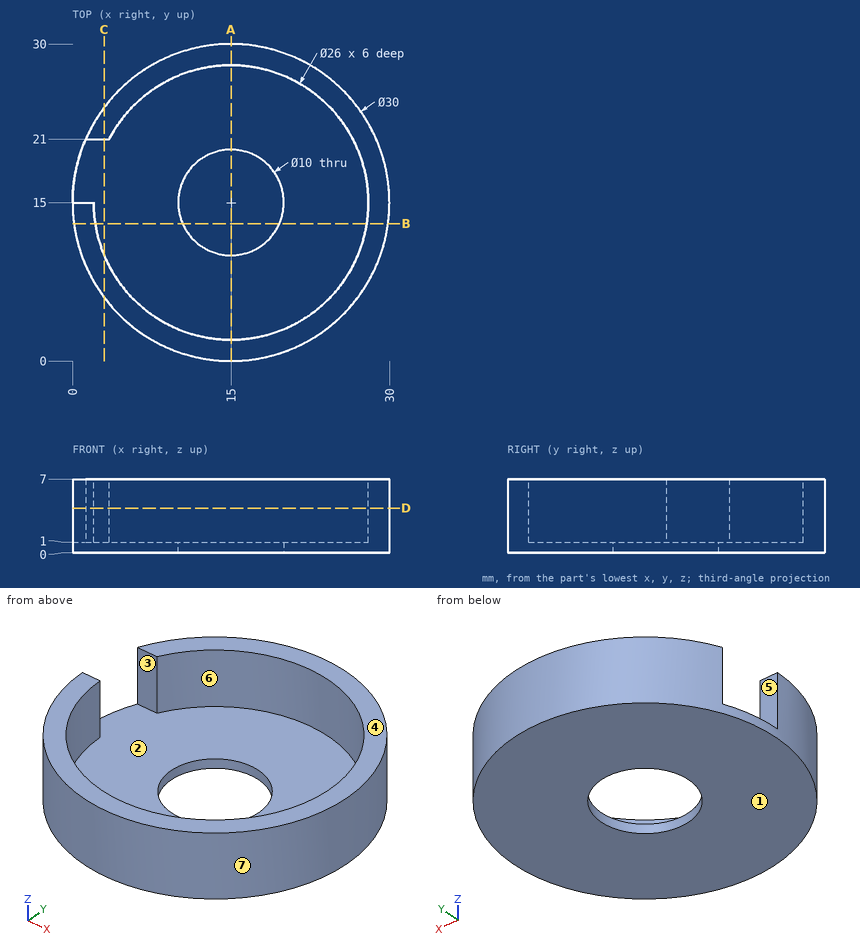
Here's the drawing with two shaded views (mm, measured from the low corner). I have some questions. A direction names the side the tool comes from. Give positions to 0.01 mm unless a question says otherwise; leave off trailing zeros. Order: outer loops, then holes, each group sorted by start corner. A loop starts at its lowest first (then second) coordinate and runs counter-clockwise, first axis right, second up. Notation, with made-up numbers: M 23,56.5 L 55,56.5 A13 ccw 55,74.5 Z; hole C -28,71.5 d8. An arc over 180 degrees is marked long. One line per question, with ' | ' between items.
Item 1: For the marked faces 1, 2 and 3, which set-ups out of +Z, -Z, +X, -X, +Y, -Y let a thin tool reach every point of the face, with its end or its side?
Answer block:
face 1: -Z, +X, -X, +Y, -Y | face 2: +Z | face 3: +Z, -X
Item 2: I'm going to push flat-ended pins straight in: pin 1 Ø1.5 at (x, z) = (13.5, 1.5) entering from -Y; pin 2 Ø6 at (x, y) = (22.5, 11.5) entering from +Z; pin 3 Ø8 at (x, y) = (8, 20.5) entering from -Z; pin 4 Ø1.6 at (x, z) = (0.5, 4.5) entering from +Y. Where does each tip first touch, or does it pass through?
Answer block:
pin 1: stops at y = 0.02 | pin 2: stops at z = 1 | pin 3: stops at z = 0 | pin 4: stops at y = 21.11
Item 3: Suppose I cut it at B-B, the plane y = 13. Write out the boundary of the cut face in (x, z), then the cut area to 3 significant figures.
Answer block:
outline: M 0.13,0 L 10.42,0 L 10.42,1 L 2.15,1 L 2.15,7 L 0.13,7 Z; M 19.58,0 L 29.87,0 L 29.87,7 L 27.85,7 L 27.85,1 L 19.58,1 Z | area: 44.8 mm2
Item 4: Suppose I cut it at A-A, the plane x = 15. Write out the boundary of the cut face in (y, z), then the cut area to 3 significant figures.
Answer block:
outline: M 0,0 L 10,0 L 10,1 L 2,1 L 2,7 L 0,7 Z; M 20,0 L 30,0 L 30,7 L 28,7 L 28,1 L 20,1 Z | area: 44.0 mm2
Item 5: We'd pull the mould along Y, two halves only. Please class the marked faces 4, 5, 6 and 7: released by +Y, released by -Y, zero draft, split by the parting line, or undercut.
Answer block:
face 4: zero draft | face 5: undercut | face 6: undercut | face 7: split by the parting line
Item 6: Suppose I cut it at D-D, the plane z = 4.25. Write out the boundary of the cut face in (x, y).
Answer block:
outline: M 0,15 A15 ccw long 1.25,21 L 3.47,21 A13 cw long 2,15 Z
Item 7: Suppose I cut it at C-C, the plane x = 3. Write out the boundary of the cut face in (y, z), then the cut area to 3 significant figures.
Answer block:
outline: M 6,0 L 24,0 L 24,7 L 21,7 L 21,1 L 10,1 L 10,7 L 6,7 Z | area: 60.0 mm2
Item 8: Please list where these lines run through material, in increasing order: L1, parallel to Y at x = 15, z = 0.55; L2, parallel to Y at x = 15, z = 2.3; L3, parallel to Z at x = 17.5, y = 27.5.
Answer block:
L1: y = 0 to 10, 20 to 30 | L2: y = 0 to 2, 28 to 30 | L3: z = 0 to 1
